from build123d import *

# Parameters (mm, degrees)
EXTRUDE2_DEPTH                  = 2.54
SKETCH5_R                       = 5.08
EXTRUDE3_DEPTH                  = 13.9446
EXTRUDE3_DEPTH_BACK             = 2.54
F_43_0_089_DIAMETER_HOLE1_D     = 2.2606
F_43_0_089_DIAMETER_HOLE1_DEPTH = 5.08
F_43_0_089_DIAMETER_HOLE1_TIP   = 0.679152758
SKETCH11_R                      = 2.95
EXTRUDE11_DEPTH                 = 17.4846
FILLET1_R                       = 1.905


with BuildPart() as part:
    # Sketch4 → Extrude2 (new body)
    with BuildSketch(Plane.XY):
        Polygon((-30.111603353, 27.840609557), (-51.701603353, 27.840609557), (-51.701603353, 22.760609557), (-50.431603353, 22.760609557), (-50.431603353, 7.520609557), (-45.351603353, 7.520609557), (-45.351603353, 22.760609557), (-30.111603353, 22.760609557), align=None)
    extrude(amount=EXTRUDE2_DEPTH)

    # Sketch5 → Extrude3 (add, two sides)
    with BuildSketch(Plane.XY.offset(2.54)) as extrude3_sk:
        with Locations((-47.891603353, 25.300609557)):
            Circle(SKETCH5_R)
    extrude(amount=EXTRUDE3_DEPTH)
    extrude(extrude3_sk.sketch, amount=-EXTRUDE3_DEPTH_BACK)

    # #43 (0.089) Diameter Hole1
    with Locations(Plane(origin=(-47.891603353, 13.281329557, 2.54), x_dir=(1, 0, 0), z_dir=(0, 0, 1))):
        with Locations((0, 0), (12.01928, 12.01928)):
            Hole(F_43_0_089_DIAMETER_HOLE1_D / 2, depth=F_43_0_089_DIAMETER_HOLE1_DEPTH)
            with Locations((0, 0, -(F_43_0_089_DIAMETER_HOLE1_DEPTH + F_43_0_089_DIAMETER_HOLE1_TIP / 2))):  # 118° drill point
                Cone(0, F_43_0_089_DIAMETER_HOLE1_D / 2, F_43_0_089_DIAMETER_HOLE1_TIP, mode=Mode.SUBTRACT)

    # Sketch11 → Extrude11 (cut, through all)
    with BuildSketch(Plane.XY.offset(16.4846)):
        with Locations((-47.891603353, 25.300609557)):
            Circle(SKETCH11_R)
    extrude(amount=-EXTRUDE11_DEPTH, mode=Mode.SUBTRACT)

    # Fillet1
    fillet1_edges = [part.edges().sort_by_distance(p)[0] for p in [
        (-30.111603353, 22.760609557, 1.27),
        (-45.351603353, 7.520609557, 1.27),
        (-50.431603353, 7.520609557, 1.27),
        (-30.111603353, 27.840609557, 1.27),
    ]]
    fillet(fillet1_edges, radius=FILLET1_R)


solid = part.part
Verification items for the finished model (mm, model axes). A direction names the side the tool comes from. Coordinates: 2 decimals unless noted, no trailing zeros. Write each loop counter-clockwise with the first axis right and the second up, starting at its lowest first coordinate (ties: lowest second). Pieces come first, ordered by that corner, then holes. Notation, with made-up numbers: M -30,79 L -11,79 A26 cw -11,112 Z; hole C -33,40 d2. An arc over 180 degrees is marked long. Use CSV: the item, a comma, the result in double quotes.
Q1. Section check C-C, the plane z = 1.5. Enter the section's corners in (x, y) (3 decimals).
Computed values:
outline,"M -50.432,9.426 A1.905 ccw -48.527,7.521 L -47.257,7.521 A1.905 ccw -45.352,9.426 L -45.352,20.901 A5.08 ccw -43.492,22.761 L -32.017,22.761 A1.905 ccw -30.112,24.666 L -30.112,25.936 A1.905 ccw -32.017,27.841 L -43.492,27.841 A5.08 ccw long -50.432,20.901 Z; hole C -47.892,25.301 d5.9; hole C -47.892,13.281 d2.261; hole C -35.872,25.301 d2.261"
Q2. Mould release check, pull along X, two halves, no side actions. Record for faces 6 (the cylindrical face through (-45.895, 8.093, 1.288)), 7 (the flat face through (-38, 22.761, 1)), 8 (the cylindrical face through (-48.97, 13.62, 1.25)): pulls with the +X half, pulls with the -X half, needs draft (parallel to the pull), parting line crosses it, or undercut.
Computed values:
face 6,"pulls with the +X half"
face 7,"needs draft"
face 8,"undercut"
Q3. Thickness scan on line 1 along X through (y, z) = (25.25, 3.25); line 2 along Y through (x, z) = (-47.75, 9); line 3 along X through (y, z) = (16.75, 2). Record the ranges inside material, lowest first. Write a range as [from, to].
Computed values:
line 1,"[-52.97, -50.84], [-44.94, -42.81]"
line 2,"[20.22, 22.35], [28.25, 30.38]"
line 3,"[-50.43, -45.35]"
Q4. Section check B-B, the plane y = 27.5. Enter the section's corners in (x, z).
Computed values:
outline,"M -52.47,0 L -49.86,0 L -49.86,16.48 L -52.47,16.48 Z; M -45.93,0 L -30.93,0 L -30.93,2.54 L -43.31,2.54 L -43.31,16.48 L -45.93,16.48 Z"
Q5. Set-up check for faces 1 (the flat face through (-48, 7.521, 1)), 2 (the flat face through (-45.7, 23.1, 16.485)), 3 (the flat face through (-38, 27.841, 1)), 4 (the flat face through (-45.352, 15, 1)), 5 (the flat face through (-50.432, 15, 1)): record each of +Z, -Z, +X, -X, +Y, -Y from which the full face is reachable in a straight line by a thin tool's end or side.
Computed values:
face 1,"+Z, -Z, +X, -X, -Y"
face 2,"+Z, +X, -X, +Y, -Y"
face 3,"+Z, -Z, +X, +Y"
face 4,"+Z, -Z, +X, -Y"
face 5,"+Z, -Z, -X, -Y"
Q6. Section check A-A, the plane x = -46.25. Enter the section's corners in (y, z), and give its area (3 significant figures).
Computed values:
outline,"M 7.81,0 L 22.85,0 L 22.85,16.48 L 20.49,16.48 L 20.49,2.54 L 7.81,2.54 Z; M 27.75,0 L 30.11,0 L 30.11,16.48 L 27.75,16.48 Z"
area,"110 mm²"
Q7. Go/stop test with flat-tipped pins: P1, Ø1, axis at x = -33, y = 24, coming from the +Z side; P2, Ø5, axis at y = 27.5, z = 5.5, coming from the -X side; P3, Ø3, axis at x = -35, z = 1.5, coming from the -Y side; P4, Ø2, axis at x = -50, z = 8.5, coming from the -Y side. Record where each tip stops, or that it passes through.
Computed values:
P1,"z = 2.54"
P2,"x = -52.97"
P3,"y = 22.76"
P4,"y = 20.34"
Q8. Section check D-D, the plane y = 15.5. Enter the section's corners in (x, z).
Computed values:
outline,"M -50.43,0 L -45.35,0 L -45.35,2.54 L -50.43,2.54 Z"
